from build123d import *

# Parameters (mm, degrees)
SKETCH_1_R          = 2
SKETCH_1_R_2        = 1.5
SKETCH_1_W          = 25
SKETCH_1_H          = 2
EXTRUDE_1_DEPTH     = 3
CUT_EXTRUDE_1_DEPTH = 124.020323524
CUT_EXTRUDE_2_DEPTH = 124.020323524
FILLET_1_R          = 2


with BuildPart() as part:
    # 草图1 → 凸台-拉伸1 (new body)
    with BuildSketch(Plane(origin=(0, 0, 0), x_dir=(1, 0, 0), z_dir=(0, 1, 0))):
        Polygon((55, 110), (55, 0), (-55, 0), (-55, 110), (-40, 110), (-40, 15), (40, 15), (40, 110), align=None)
        with Locations(Location((47.5, 32.5, 0), (0, 0, 270))):
            Circle(SKETCH_1_R, mode=Mode.SUBTRACT)
        with Locations(Location((47.5, 7.5, 0), (0, 0, 270))):
            Circle(SKETCH_1_R, mode=Mode.SUBTRACT)
        with Locations(Location((47.5, 79.5, 0), (0, 0, 270))):
            Circle(SKETCH_1_R, mode=Mode.SUBTRACT)
        with Locations(Location((47.5, 102.5, 0), (0, 0, 270))):
            Circle(SKETCH_1_R, mode=Mode.SUBTRACT)
        with Locations(Location((-47.5, 102.5, 0), (0, 0, 90))):
            Circle(SKETCH_1_R, mode=Mode.SUBTRACT)
        with Locations(Location((-47.5, 79.5, 0), (0, 0, 90))):
            Circle(SKETCH_1_R, mode=Mode.SUBTRACT)
        with Locations(Location((-47.5, 7.5, 0), (0, 0, 90))):
            Circle(SKETCH_1_R, mode=Mode.SUBTRACT)
        with Locations(Location((-47.5, 32.5, 0), (0, 0, 90))):
            Circle(SKETCH_1_R, mode=Mode.SUBTRACT)
        with Locations(Location((17.5, 5, 0), (0, 0, 270))):
            Circle(SKETCH_1_R_2, mode=Mode.SUBTRACT)
        with Locations(Location((-17.5, 5, 0), (0, 0, 90))):
            Circle(SKETCH_1_R_2, mode=Mode.SUBTRACT)
        with Locations((0, 11)):
            Rectangle(SKETCH_1_W, SKETCH_1_H, mode=Mode.SUBTRACT)
    extrude(amount=EXTRUDE_1_DEPTH)

    # 草图2 → 切除-拉伸1 (cut, through all)
    with BuildSketch(Plane(origin=(0, 3, 0), x_dir=(1, 0, 0), z_dir=(0, 1, 0))):
        with BuildLine():
            Line((-12.5, 10), (-10.5, 10))
            ThreePointArc((-10.5, 10), (-11.5, 9), (-12.5, 10))
        make_face()
        with BuildLine():
            Line((12.5, 12), (10.5, 12))
            ThreePointArc((10.5, 12), (11.5, 13), (12.5, 12))
        make_face()
        with BuildLine():
            Line((-10.5, 12), (-12.5, 12))
            ThreePointArc((-12.5, 12), (-11.5, 13), (-10.5, 12))
        make_face()
        with BuildLine():
            Line((10.5, 10), (12.5, 10))
            ThreePointArc((12.5, 10), (11.5, 9), (10.5, 10))
        make_face()
    extrude(amount=-CUT_EXTRUDE_1_DEPTH, mode=Mode.SUBTRACT)

    # 草图3 → 切除-拉伸2 (cut, through all)
    with BuildSketch(Plane(origin=(0, 3, 0), x_dir=(1, 0, 0), z_dir=(0, 1, 0))):
        with BuildLine():
            Line((-45.5, 70), (-45.5, 42))
            ThreePointArc((-45.5, 42), (-47.5, 40), (-49.5, 42))
            Line((-49.5, 42), (-49.5, 70))
            ThreePointArc((-49.5, 70), (-47.5, 72), (-45.5, 70))
        make_face()
        with BuildLine():
            Line((45.5, 70), (45.5, 42))
            ThreePointArc((45.5, 42), (47.5, 40), (49.5, 42))
            Line((49.5, 42), (49.5, 70))
            ThreePointArc((49.5, 70), (47.5, 72), (45.5, 70))
        make_face()
    extrude(amount=-CUT_EXTRUDE_2_DEPTH, mode=Mode.SUBTRACT)

    # 圆角1
    fillet_1_edges = [part.edges().sort_by_distance(p)[0] for p in [
        (55, 1.5, -110),
        (55, 1.5, 0),
        (-55, 1.5, 0),
        (-55, 1.5, -110),
        (-40, 1.5, -110),
        (-40, 1.5, -15),
        (40, 1.5, -15),
        (40, 1.5, -110),
    ]]
    fillet(fillet_1_edges, radius=FILLET_1_R)


solid = part.part
Model file for the job. Use its own axes, mm. A direction names the side the tool comes from. Give positions to 0.01 mm unless a question says otherwise; leave off trailing zeros. Write each loop counter-clockwise with the first axis right and the second up, starting at its lowest first coordinate (ties: lowest second). Pieces come first, ordered by that corner, then holes. Notation, with made-up numbers: M 21.25,85 L 66.25,85 A10 ccw 66.25,95 Z; hole C 9,77 d11. An arc over 180 degrees is marked long. One line per item, written item: value. Start each with the question number.
Q1. Saw through at C-C, the plane x = -47.5. Write the cut outline in (y, z), plus the area to 3 significant figures.
Q2. Two-plate mould, pull along Z, no slides. Class faces 4 (the flat face through (-48, 1, -110)), 5 (the flat face through (55, 1, -56)), 6 (the flat face through (0, 1, -12)): +Z half, -Z half, draft (parallel to the pull), parting line (faces both ways), or undercut.
Q3. Saw through at D-D, the plane y = 1.15. State how many separate pieces and enclosed holes the cut face has, plus the area to 3 significant figures.
Q4. Saw through at A-A, the plane z = -102.5. Write the cut outline in (x, y).
Q5. 3-axis set-ups, long thin cutter, end or side, ignore diameter. For faces 1 (the flat face through (-55, 1, -54)), 2 (the flat face through (-1, 1, -15)), 3 (the flat face through (-45.5, 2, -56)): which of +Z, -Z, +X, -X, +Y, -Y reach the whole face in a straight line?
Q6. Drop a flat-ended pin along its axis: pin 1 Ø1.5 at (x, y) = (-14.5, 1.5) entering from -Z. Give the stop position or say it passes through.
Q7. Saw through at B-B, the plane z = -23. Write the cut outline in (x, y).
Q8. Probe probe 1 along X at (y, z) = (1.8, -7.5); probe 2 along X at (y, z) = (0.7, -32.5); probe 3 along Z at (x, y) = (-47.5, 1.1). List the from-to ranges inside material, lowest first. Write a range as [from, to].
Output values:
1. outline: M 0,-110 L 3,-110 L 3,-104.5 L 0,-104.5 Z; M 0,-100.5 L 3,-100.5 L 3,-81.5 L 0,-81.5 Z; M 0,-77.5 L 3,-77.5 L 3,-72 L 0,-72 Z; M 0,-40 L 3,-40 L 3,-34.5 L 0,-34.5 Z; M 0,-30.5 L 3,-30.5 L 3,-9.5 L 0,-9.5 Z; M 0,-5.5 L 3,-5.5 L 3,0 L 0,0 Z
1. area: 186 mm²
2. face 4: -Z half
2. face 5: draft
2. face 6: undercut
3. separate pieces: 1
3. enclosed holes: 13
3. area: 4,080 mm²
4. outline: M -55,0 L -49.5,0 L -49.5,3 L -55,3 Z; M -45.5,0 L -40,0 L -40,3 L -45.5,3 Z; M 40,0 L 45.5,0 L 45.5,3 L 40,3 Z; M 49.5,0 L 55,0 L 55,3 L 49.5,3 Z
5. face 1: +Z, -Z, -X, +Y, -Y
5. face 2: -Z, +Y, -Y
5. face 3: +Y, -Y
6. pin 1: stops at z = -15
7. outline: M -55,0 L -40,0 L -40,3 L -55,3 Z; M 40,0 L 55,0 L 55,3 L 40,3 Z
8. probe 1: x = [-55, -49.5], [-45.5, 45.5], [49.5, 55]
8. probe 2: x = [-55, -49.5], [-45.5, -40], [40, 45.5], [49.5, 55]
8. probe 3: z = [-110, -104.5], [-100.5, -81.5], [-77.5, -72], [-40, -34.5], [-30.5, -9.5], [-5.5, 0]
